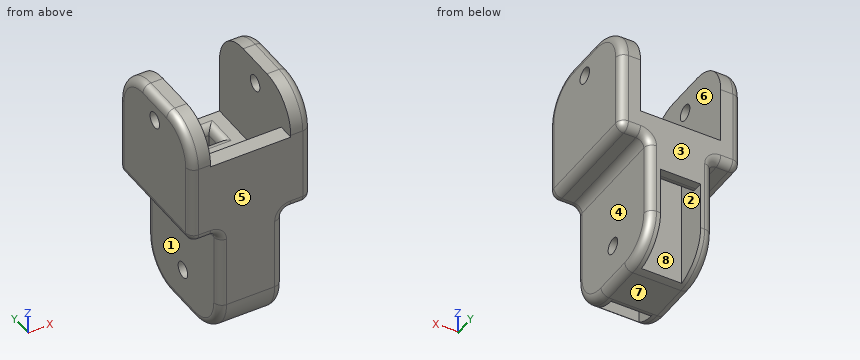
from build123d import *

# Parameters (mm, degrees)
BASE_SKETCH_W                    = 15
BASE_SKETCH_H                    = 15
BASE_SKETCH_EXTRUDE_DEPTH        = 30
CENTER_NUB_CUTOUT_SKETCH_W       = 3.5
CENTER_NUB_CUTOUT_SKETCH_H       = 15
HINGE_NUB_EXTRUDED_CUT_DEPTH     = 15
HINGE_CUTOUT_SKETCH_W            = 10
HINGE_CUTOUT_SKETCH_H            = 15
HINGE_CUTOUT_EXTRUDED_CUT_DEPTH  = 12
HINGE_HOLE_SKETCH_R              = 1
HINGE_HOLE_EXTRUDED_CUT_DEPTH    = 35.369317712
CORNER_FILLETS_R                 = 5
STYLE_FILLETS_R                  = 1
ROUTING_HOLES_SKETCH_W           = 5
ROUTING_HOLES_SKETCH_H           = 2
ROUTING_HOLES_EXTRUDED_CUT_DEPTH = 32.819805153
SKETCH1_W                        = 10
SKETCH1_H                        = 2
BACKING_EXTRUDE_DEPTH            = 6.75
EXTRA_ROUTING_CUT_SKETCH_W       = 5
EXTRA_ROUTING_CUT_SKETCH_H       = 10
EXTRA_ROUTING_EXTRUDED_CUT_DEPTH = 4
ROUTING_FILLETS_R                = 1


with BuildPart() as part:
    # Base Sketch → Base Sketch Extrude (new body)
    with BuildSketch(Plane.XY):
        Rectangle(BASE_SKETCH_W, BASE_SKETCH_H)
    extrude(amount=BASE_SKETCH_EXTRUDE_DEPTH)

    # Center Nub Cutout Sketch → Hinge Nub Extruded Cut (cut)
    with BuildSketch(Plane.XY):
        with Locations((5.75, 0)):
            Rectangle(CENTER_NUB_CUTOUT_SKETCH_W, CENTER_NUB_CUTOUT_SKETCH_H)
        with Locations((-5.75, 0)):
            Rectangle(CENTER_NUB_CUTOUT_SKETCH_W, CENTER_NUB_CUTOUT_SKETCH_H)
    extrude(amount=HINGE_NUB_EXTRUDED_CUT_DEPTH, mode=Mode.SUBTRACT)

    # Hinge Cutout Sketch → Hinge Cutout Extruded Cut (cut)
    with BuildSketch(Plane.XY.offset(30)):
        Rectangle(HINGE_CUTOUT_SKETCH_W, HINGE_CUTOUT_SKETCH_H)
    extrude(amount=-HINGE_CUTOUT_EXTRUDED_CUT_DEPTH, mode=Mode.SUBTRACT)

    # Hinge Hole Sketch → Hinge Hole Extruded Cut (cut, through all)
    with BuildSketch(Plane(origin=(7.5, 0, 0), x_dir=(0, 0, -1), z_dir=(1, 0, 0))):
        with Locations(Location((-5, 0, 0), (0, 0, 90))):
            Circle(HINGE_HOLE_SKETCH_R)
        with Locations(Location((-27, 0, 0), (0, 0, 90))):
            Circle(HINGE_HOLE_SKETCH_R)
    extrude(amount=-HINGE_HOLE_EXTRUDED_CUT_DEPTH, mode=Mode.SUBTRACT)

    # Corner Fillets
    corner_fillets_edges = [part.edges().sort_by_distance(p)[0] for p in [
        (0, -7.5, 0),
        (0, 7.5, 0),
        (-6.25, -7.5, 30),
        (-6.25, 7.5, 30),
        (6.25, -7.5, 30),
        (6.25, 7.5, 30),
    ]]
    fillet(corner_fillets_edges, radius=CORNER_FILLETS_R)

    # Style Fillets
    style_fillets_edges = [part.edges().sort_by_distance(p)[0] for p in [
        (4, 7.5, 10),
        (4, -7.5, 10),
        (7.5, 0, 15),
        (5.75, 7.5, 15),
        (4, 0, 15),
        (5.75, -7.5, 15),
        (-4, -7.5, 10),
        (-4, 7.5, 10),
        (-7.5, 0, 15),
        (-5.75, -7.5, 15),
        (-4, 0, 15),
        (-5.75, 7.5, 15),
        (-7.5, 0, 30),
        (-7.5, -7.5, 20),
        (7.5, -7.5, 20),
        (-7.5, 7.5, 20),
        (-7.5, 6.035533906, 28.535533906),
        (-7.5, -6.035533906, 28.535533906),
        (7.5, 7.5, 20),
        (7.5, 0, 30),
        (7.5, 6.035533906, 28.535533906),
        (7.5, -6.035533906, 28.535533906),
        (4, 0, 0),
        (4, 6.035533906, 1.464466094),
        (4, -6.035533906, 1.464466094),
        (-4, 0, 0),
        (-4, 6.035533906, 1.464466094),
        (-4, -6.035533906, 1.464466094),
    ]]
    fillet(style_fillets_edges, radius=STYLE_FILLETS_R)

    # Routing Holes Sketch → Routing Holes Extruded Cut (cut, through all)
    with BuildSketch(Plane.XY):
        with Locations((0, 4.5)):
            Rectangle(ROUTING_HOLES_SKETCH_W, ROUTING_HOLES_SKETCH_H)
        with Locations((0, -4.5)):
            Rectangle(ROUTING_HOLES_SKETCH_W, ROUTING_HOLES_SKETCH_H)
    extrude(amount=ROUTING_HOLES_EXTRUDED_CUT_DEPTH, mode=Mode.SUBTRACT)

    # Sketch1 → Backing Extrude (add)
    with BuildSketch(Plane.XY.offset(18)):
        with Locations((0, -6.5)):
            Rectangle(SKETCH1_W, SKETCH1_H)
    extrude(amount=BACKING_EXTRUDE_DEPTH)

    # Extra Routing Cut Sketch → Extra Routing Extruded Cut (cut)
    with BuildSketch(Plane(origin=(0, 7.5, 0), x_dir=(1, 0, 0), z_dir=(0, 1, 0))):
        with Locations((0, -6)):
            Rectangle(EXTRA_ROUTING_CUT_SKETCH_W, EXTRA_ROUTING_CUT_SKETCH_H)
    extrude(amount=-EXTRA_ROUTING_EXTRUDED_CUT_DEPTH, mode=Mode.SUBTRACT)

    # Routing Fillets
    routing_fillets_edges = [part.edges().sort_by_distance(p)[0] for p in [
        (0, -3.5, 0.101020514),
        (-2.5, 4.5, 18),
        (0, 3.5, 18),
        (2.5, 4.5, 18),
        (0, 5.5, 18),
        (2.5, -4.5, 18),
        (0, -3.5, 18),
        (-2.5, -4.5, 18),
        (0, 5.5, 11),
    ]]
    fillet(routing_fillets_edges, radius=ROUTING_FILLETS_R - 0.0001)  # a hair under: the kernel refuses the full size


solid = part.part
For this review, take the finished solid that the model builds, in its own axes (mm). Face numbers are marked on the shaded views. A direction names the side the tool comes from. Round coordinates to 2 decimals unless told otherwise and drop trailing zeros. Order: outer loops, then holes, each group sorted by start corner. A loop starts at its lowest first (then second) coordinate and runs counter-clockwise, first axis right, second up. Notation, with made-up numbers: (-39.5, 9.5) -> (-16.5, 9.5) arc R10 ccw to (-16.5, 17.5) -> close; hole circle Ø9 at (-37.75, -34). An arc over 180 degrees is marked (long way). Put each result on its own line as item: value.
Q1. Add section A-A on x = -2. State how many separate pieces and enclosed holes the cut face has, plus the area to 3 significant figures.
Check result:
separate pieces: 3
enclosed holes: 1
area: 181 mm2
Q2. Insertion check: pin 1 Ø6 at (y, z) = (-5, 9) entering from -X; pin 2 Ø1.2 at (x, y) = (6, -3) entering from -Z; pin 3 Ø1.5 at (x, y) = (-1, -2) entering from +Z. Each pin has a flat end and moves straight along its axis. Give the tip position at first contact, or say it passes through.
Check result:
pin 1: x = -4
pin 2: z = 15
pin 3: z = 18
Q3. For probe 1 along X at (y, z) = (-1.75, 27.75); probe 2 along Y at (x, z) = (0.25, 8.25); probe 3 along Y at (x, z) = (4.5, 22.25), list the stretches that pass through material, from the lowest coordinate up. Write a range as [from, to].
Check result:
probe 1: [-7.5, -5], [5, 7.5]
probe 2: [-7.5, -5.5], [-3.5, 3.5]
probe 3: [-7.5, -5.5]
Q4. Add section C-C on z = 7.75. Write out the cut boundary in (x, y), plus the area to 3 significant figures.
Check result:
outline: (-4, -6.5) arc R1 ccw to (-3, -7.5) -> (3, -7.5) arc R1 ccw to (4, -6.5) -> (4, 6.5) arc R1 ccw to (3, 7.5) -> (2.5, 7.5) -> (2.5, 3.5) -> (-2.5, 3.5) -> (-2.5, 7.5) -> (-3, 7.5) arc R1 ccw to (-4, 6.5) -> close; hole (-2.5, -5.5) -> (2.5, -5.5) -> (2.5, -3.5) -> (-2.5, -3.5) -> close
area: 89.1 mm2
Q5. Machinability: for the marked faces 4, 5, 6, 7 and 8, which of the approach directions +Z, -Z, +X, -X, +Y, -Y give a long, thin tool a straight path to every point of the face, cutting with its end or side? Answer none if there is none.
Check result:
face 4: -Z, +X, +Y, -Y
face 5: +Z, -Z, +X, -X, -Y
face 6: +Z, +Y
face 7: -Z, +X, -X, +Y, -Y
face 8: +Z, -Z
Q6. Add section D-D on y = 1.75. Write out the cut boundary in (x, z), plus the area to 3 significant figures.
Check result:
outline: (-7.5, 16) arc R1 ccw to (-6.5, 15) -> (-5, 15) arc R1 cw to (-4, 14) -> (-4, 1) arc R1 ccw to (-3, 0) -> (3, 0) arc R1 ccw to (4, 1) -> (4, 14) arc R1 cw to (5, 15) -> (6.5, 15) arc R1 ccw to (7.5, 16) -> (7.5, 29) arc R1 ccw to (6.5, 30) -> (5, 30) -> (5, 18) -> (-5, 18) -> (-5, 30) -> (-6.5, 30) arc R1 ccw to (-7.5, 29) -> close
area: 224 mm2
Q7. Mouldability with a two-part tool opening along X and no side actions: class the marked faces 1, 2 and 3 as pulls with the +X half, pulls with the -X half, needs draft (parallel to the pull), parting line crosses it, or undercut.
Check result:
face 1: pulls with the -X half
face 2: undercut
face 3: needs draft
